Check sheet for the modelled part. Datum: model origin and axes. Units: mm. Face numbers are marked on the shaded views. A direction names the side the tool comes from. Give positions to 0.01 mm unless a question says otherwise; leave off trailing zeros. Write each loop counter-clockwise with the first axis right and the second up, starting at its lowest first coordinate (ties: lowest second). Pieces come first, ordered by that corner, then holes. Notation, with made-up numbers: (31.25, 68.5) -> (61.25, 68.5) arc R17 ccw to (61.25, 92.5) -> close; hole circle Ø8 at (11, 23). An arc over 180 degrees is marked (long way). Use a Markdown table: item, result. Add a question column.
1. Cross-section at C-C (x = -26). Enter the section's corners in (y, z).
2. Set-up check for the marked faces 1, 2, 3, 4 and 5: record each of +Z, -Z, +X, -X, +Y, -Y from which the full face is reachable in a straight line by a thin tool's end or side.
3. Release check for a two-part mould opening along X. For the marked faces 6, 7 and 8 record: released by +X, released by -X, zero draft, split by the parting line, or undercut.
4. Cross-section at A-A (y = -9.5). Enter the section's corners in (x, z), then the cut area to 3 significant figures.
5. Cross-section at B-B (x = 10.5). Enter the section's corners in (y, z), then the cut area to 3 significant figures.
6. Scan lines: probe 1 along X at (y, z) = (-2, 2); probe 2 along X at (y, z) = (10, 0.75); probe 3 along X at (y, z) = (-9, 4.75). Record each from-to range of solid material in increasing order. Write a range as [from, to].
7. Gauge pin test, flat ends, axial feed: P1, Ø1, axis at y = 13.5, z = 3, coming from the -X side; P2, Ø1.4, axis at y = 7, z = 2.5, coming from the +X side; P3, Ø2, axis at x = -4.5, y = 12, coming from the +Z side. Record the tip position at first contact, or that the pin passes through.
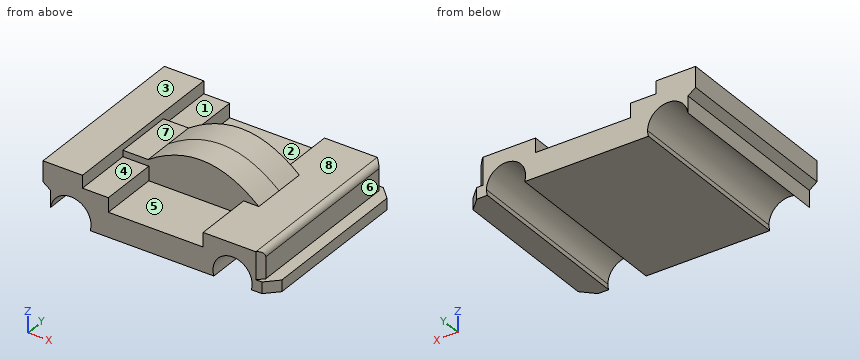
from build123d import *

# Parameters (mm, degrees)
F1_DEPTH = 19.05
F2_DEPTH = 6.35
F3_DEPTH = 6.35
F4_SIZE  = 2.54
F5_SIZE  = 1.27
F6_R     = 1.27


with BuildPart() as f1:
    # F0 (on Front) → F1 (new body, symmetric)
    with BuildSketch(Plane.XZ):
        with BuildLine():
            Line((-24.059453, 8.571546), (-32.558522, 8.571546))
            Line((-32.558522, 8.571546), (-32.558522, 4.165861))
            Line((-32.558522, 4.165861), (-30.917545, 2.935127))
            Line((-30.917545, 2.935127), (-30.917545, 0))
            Line((-30.917545, 0), (-30.917545, -0.634123))
            ThreePointArc((-30.917545, -0.634123), (-26.288961, 3.138165), (-22.212116, -1.224549))
            ThreePointArc((-22.212116, -1.224549), (-22.257831, -1.855194), (-22.394021, -2.472653))
            Line((-22.394021, -2.472653), (4.261856, -2.472653))
            ThreePointArc((4.261856, -2.472653), (7.65477, 2.941104), (12.499143, -1.224549))
            ThreePointArc((12.499143, -1.224549), (12.451597, -1.855724), (12.310032, -2.472653))
            Line((12.310032, -2.472653), (17.1531, -2.472653))
            Line((17.1531, -2.472653), (17.1531, -0.025919))
            Line((17.1531, -0.025919), (14.57005, -0.025919))
            Line((14.57005, -0.025919), (14.57005, 0))
            Line((14.57005, 0), (14.57005, 5.856519))
            Line((14.57005, 5.856519), (10.009351, 5.856519))
            Line((10.009351, 5.856519), (5.226919, 5.856519))
            Line((5.226919, 5.856519), (1.940277, 5.856519))
            Line((1.940277, 5.856519), (1.940277, 2.793992))
            Line((1.940277, 2.793992), (-18.475659, 2.793992))
            Line((-18.475659, 2.793992), (-18.475659, 5.856519))
            Line((-18.475659, 5.856519), (-18.621231, 5.856519))
            Line((-18.621231, 5.856519), (-24.059453, 5.856519))
            Line((-24.059453, 5.856519), (-24.059453, 6.833025))
            Line((-24.059453, 6.833025), (-24.059453, 7.214033))
            Line((-24.059453, 7.214033), (-24.059453, 8.571546))
        make_face()
    extrude(amount=F1_DEPTH, both=True)

    # F0 (on Front) → F2 (join, symmetric)
    with BuildSketch(Plane.XZ):
        with BuildLine():
            add(Edge.make_bspline(
                [(-18.621231, 7.214033), (-9.229071, 13.654015), (-1.348382, 11.55533), (5.226919, 5.856519)],
                knots=[0, 0, 0, 0, 23.886756, 23.886756, 23.886756, 23.886756], degree=3))
            Line((-18.621231, 7.214033), (-18.621231, 5.856519))
            Line((-18.621231, 5.856519), (-18.475659, 5.856519))
            Line((-18.475659, 5.856519), (-18.475659, 2.793992))
            Line((-18.475659, 2.793992), (1.940277, 2.793992))
            Line((1.940277, 2.793992), (1.940277, 5.856519))
            Line((1.940277, 5.856519), (5.226919, 5.856519))
        make_face()
    extrude(amount=F2_DEPTH, both=True)

    # F0 (on Front) → F3 (join, symmetric)
    with BuildSketch(Plane.XZ):
        Polygon((-18.621231, 7.214033), (-24.059453, 7.214033), (-24.059453, 6.833025), (-24.059453, 5.856519), (-18.621231, 5.856519), align=None)
    extrude(amount=F3_DEPTH, both=True)

    # F4
    f4_edges = [f1.edges().sort_by_distance(p)[0] for p in [
        (17.1531, -19.05, -1.249286),
        (17.1531, 19.05, -1.249286),
    ]]
    chamfer(f4_edges, length=F4_SIZE)

    # F5
    f5_edges = [f1.edges().sort_by_distance(p)[0] for p in [
        (14.57005, -19.05, 2.9153),
        (14.57005, 19.05, 2.9153),
    ]]
    chamfer(f5_edges, length=F5_SIZE)

    # F6
    f6_edges = [f1.edges().sort_by_distance(p)[0] for p in [
        (14.57005, 0, 5.856519),
    ]]
    fillet(f6_edges, radius=F6_R)


solid = f1.part
Worked answers:
| question | item | result |
|---|---|---|
| 1 | outline | (-19.05, 3.11) -> (19.05, 3.11) -> (19.05, 8.57) -> (-19.05, 8.57) -> close |
| 2 | face 1 | +Z, +X, +Y |
| 2 | face 2 | +Z, +Y |
| 2 | face 3 | +Z, -X, +Y, -Y |
| 2 | face 4 | +Z, +X, -Y |
| 2 | face 5 | +Z, -Y |
| 3 | face 6 | released by +X |
| 3 | face 7 | undercut |
| 3 | face 8 | zero draft |
| 4 | outline | (-32.56, 4.17) -> (-30.92, 2.94) -> (-30.92, -0.63) arc R4.37 cw to (-22.21, -1.22) arc R4.37 cw to (-22.39, -2.47) -> (4.26, -2.47) arc R4.21 cw (long way) to (12.31, -2.47) -> (17.15, -2.47) -> (17.15, -0.03) -> (14.57, -0.03) -> (14.57, 4.59) arc R1.27 ccw to (13.3, 5.86) -> (1.94, 5.86) -> (1.94, 2.79) -> (-18.48, 2.79) -> (-18.48, 5.86) -> (-24.06, 5.86) -> (-24.06, 8.57) -> (-32.56, 8.57) -> close |
| 4 | area | 270 mm² |
| 5 | outline | (-19.05, 2.36) -> (19.05, 2.36) -> (19.05, 5.86) -> (-19.05, 5.86) -> close |
| 5 | area | 133 mm² |
| 6 | probe 1 | x = [-30.92, -29.54], [-23.63, 5.57], [11, 14.57] |
| 6 | probe 2 | x = [-30.92, -30.49], [-22.68, 4.56], [12.01, 14.57] |
| 6 | probe 3 | x = [-32.56, -18.48], [1.94, 14.56] |
| 7 | P1 | stops at x = -31.67 |
| 7 | P2 | stops at x = 14.57 |
| 7 | P3 | stops at z = 2.79 |
